Part model, mm, in its own coordinate system. A direction names the side the tool comes from. Round coordinates to 2 decimals unless told otherwise and drop trailing zeros. Write each loop counter-clockwise with the first axis right and the second up, starting at its lowest first coordinate (ties: lowest second). Pieces come first, ordered by that corner, then holes. Notation, with made-up numbers: M 4.5,44.25 L 51.5,44.25 A14 ccw 51.5,61.25 Z; hole C 45.5,-14 d11. An arc over 180 degrees is marked long. Use a Markdown table: item, result. Add a question column.
1) Two-plate mould, pull along Z, no slides. Class faces 5 (the face through (-0.04, -10, 137.17)), 6 (the face through (-0.063, -5.105, 127.525)), 7 (the face through (0.192, -0.865, 84.782)): released by +Z, released by -Z, zero draft, split by the parting line, or undercut.
2) Wall check: probe 1 along Z at (x, y) = (0, 5.75); probe 2 along Z at (x, y) = (-12.5, -2.75); probe 3 along Y at (x, z) = (0, 64). Give the ranges that are in metal, low to high.
3) Slice it at A-A on x = -9.75. Write the cut outline in (y, z), plus the area to 3 significant figures.
4) Slice it at D-D on z = 132. Write the cut outline in (x, y), plus the area to 3 significant figures.
5) Which spindle directions (+Z, -Z, +X, -X, +Y, -Y) get a long thin tool onto all of the face, cutting with end or side? Do faces 1 (the face through (0.093, 9.995, 137.169)), 2 (the face through (2.4, -4.5, 41.7)), 3 (the face through (-4.5, 0, 139)), 4 (the face through (-9.1, 9.1, 114.5)). Say none if no direction does.
6) Slice it at C-C on z = 87. Write the cut outline in (x, y).
7) Slice it at B-B on z = 26. Write the cut outline in (x, y).
8) Drop flat-ended pins along their axis: P1, Ø1.5, axis at x = 1.5, z = 75, coming from the -Y side; P2, Ø12, axis at y = -8, z = 139.5, coming from the +X side; P3, Ø2, axis at x = 6, z = 67, coming from the -Y side (3 decimals); P4, Ø4, axis at y = 2, z = 151.91, coming from the -X side. Give the stop position or say it passes through.
```python
from build123d import *

# Parameters (mm, degrees)
SKETCH_1_R               = 13.7
EXTRUDE_1_DEPTH          = 117
SKETCH_6_W               = 1
SKETCH_6_H               = 1.5
HOLE_WIZARD_M12_1_D      = 10.2
HOLE_WIZARD_M12_1_DEPTH  = 82.25
HOLE_WIZARD_M12_1_TIP    = 3.064389157
SKETCH_9_R               = 10
EXTRUDE_3_DEPTH          = 42.91
CUT_EXTRUDE_1_DEPTH      = 162.079446547
CUT_EXTRUDE_1_DEPTH_BACK = 162.079446547
SKETCH_8_W               = 42.91
SKETCH_8_H               = 10.443945465
CHAMFER_1_SIZE           = 2
HOLE_WIZARD_7_0_7_1_D    = 7
HOLE_WIZARD_M2_1_REACH   = 164.236
HOLE_WIZARD_M2_1_BORE_R  = 0.8


with BuildPart() as part:
    # 草图1 → 凸台-拉伸1 (new body)
    with BuildSketch(Plane.XY):
        Circle(SKETCH_1_R)
    extrude(amount=EXTRUDE_1_DEPTH)

    # 草图6 → 切除-旋转1 (revolve, cut)
    with BuildSketch(Plane(origin=(0, 0, 0), x_dir=(1, 0, 0), z_dir=(0, 1, 0))):
        with Locations((-13.2, -115.25)):
            Rectangle(SKETCH_6_W, SKETCH_6_H)
    revolve(axis=Axis((0, 0, 0), (0, 0, 1)), mode=Mode.SUBTRACT)

    # M12 螺纹孔1
    with Locations(Plane(origin=(0, 0, 0), x_dir=(-1, 0, 0), z_dir=(0, 0, -1))):
        with Locations((0, 0)):
            Hole(HOLE_WIZARD_M12_1_D / 2, depth=HOLE_WIZARD_M12_1_DEPTH)
            with Locations((0, 0, -(HOLE_WIZARD_M12_1_DEPTH + HOLE_WIZARD_M12_1_TIP / 2))):  # 118° drill point
                Cone(0, HOLE_WIZARD_M12_1_D / 2, HOLE_WIZARD_M12_1_TIP, mode=Mode.SUBTRACT)

    # 草图9 → 凸台-拉伸3 (add)
    with BuildSketch(Plane.XY.offset(117)):
        with Locations((-0.231058247, 0)):
            Circle(SKETCH_9_R)
    extrude(amount=EXTRUDE_3_DEPTH)

    # 草图8 → 切除-拉伸1 (cut, two sides: drawn at the far end of the back side and taken through both)
    with BuildSketch(Plane(origin=(0, 0, 0), x_dir=(0, 0, -1), z_dir=(0, 1, 0)).offset(-CUT_EXTRUDE_1_DEPTH_BACK)):
        with Locations((-138.455, 9.721972732)):
            Rectangle(SKETCH_8_W, SKETCH_8_H)
        with Locations((-138.455, -9.721972732)):
            Rectangle(SKETCH_8_W, SKETCH_8_H)
    extrude(amount=CUT_EXTRUDE_1_DEPTH + CUT_EXTRUDE_1_DEPTH_BACK, mode=Mode.SUBTRACT)

    # 倒角1
    chamfer_1_edges = [part.edges().sort_by_distance(p)[0] for p in [
        (0.027699329, -9.996651665, 159.91),
        (0.027699329, 9.996651665, 159.91),
    ]]
    chamfer(chamfer_1_edges, length=CHAMFER_1_SIZE)

    # Ø7.0 (7) 直径孔1 (through all)
    with Locations(Plane(origin=(4.5, 0, 0), x_dir=(0, 0, -1), z_dir=(1, 0, 0))):
        with Locations((-125.91, -2), (-151.91, 2)):
            Hole(HOLE_WIZARD_7_0_7_1_D / 2)

    # M2 螺纹孔1 bore → M2 螺纹孔1 (cut, up to next)
    with BuildSketch(Plane(origin=(0, 10, 0), x_dir=(1, 0, 0), z_dir=(0, 1, 0)), mode=Mode.PRIVATE) as hole_wizard_m2_1_sk1:
        with Locations((0, -151.91)):
            Circle(HOLE_WIZARD_M2_1_BORE_R)
    hole_wizard_m2_1_tool1 = extrude(hole_wizard_m2_1_sk1.sketch, amount=-HOLE_WIZARD_M2_1_REACH, mode=Mode.PRIVATE) & part.part
    # M2 螺纹孔1 bore → M2 螺纹孔1 (cut, up to next)
    with BuildSketch(Plane(origin=(0, 10, 0), x_dir=(1, 0, 0), z_dir=(0, 1, 0)), mode=Mode.PRIVATE) as hole_wizard_m2_1_sk2:
        with Locations((0, -125.91)):
            Circle(HOLE_WIZARD_M2_1_BORE_R)
    hole_wizard_m2_1_tool2 = extrude(hole_wizard_m2_1_sk2.sketch, amount=-HOLE_WIZARD_M2_1_REACH, mode=Mode.PRIVATE) & part.part
    add(hole_wizard_m2_1_tool1.solids().sort_by_distance((0, 10, 151.91))[0], mode=Mode.SUBTRACT)
    add(hole_wizard_m2_1_tool2.solids().sort_by_distance((0, 10, 125.91))[0], mode=Mode.SUBTRACT)


solid = part.part
```
Entries:
| question | item | result |
|---|---|---|
| 1 | face 5 | zero draft |
| 1 | face 6 | undercut |
| 1 | face 7 | released by -Z |
| 2 | probe 1 | z = 0 to 125.11, 126.71 to 151.11, 152.71 to 159.91 |
| 2 | probe 2 | z = 0 to 114.5, 116 to 117 |
| 2 | probe 3 | y = -13.7 to -5.1, 5.1 to 13.7 |
| 3 | outline | M -9.62,0 L 9.62,0 L 9.62,114.5 L 8.14,114.5 L 8.14,116 L 9.62,116 L 9.62,117 L -9.62,117 L -9.62,116 L -8.14,116 L -8.14,114.5 L -9.62,114.5 Z |
| 3 | area | 2,250 mm^2 |
| 4 | outline | M -4.5,-9.04 A10 ccw 4.5,-8.81 L 4.5,8.81 A10 ccw -4.5,9.04 Z |
| 4 | area | 174 mm^2 |
| 5 | face 1 | +Z, +Y |
| 5 | face 2 | -Z |
| 5 | face 3 | +Z, -X, +Y, -Y |
| 5 | face 4 | none |
| 6 | outline | C 0,0 d27.4 |
| 7 | outline | C 0,0 d27.4; hole C 0,0 d10.2 |
| 8 | P1 | stops at y = -13.68 |
| 8 | P2 | stops at x = 4.5 |
| 8 | P3 | stops at y = -12.755 |
| 8 | P4 | passes through |
